```python
from build123d import *

# Parameters (mm, degrees)
F2_DEPTH = 2


# Not quite as in the source:
# - the program builds the solid bodies; features that only make, move or delete a surface that nothing else refers to are left out


with BuildPart() as f2:
    # F0 (on Top) → F2 (new body)
    with BuildSketch(Plane.XY):
        Polygon((-350, -225), (350, -225), (350, -217.2532975674), (350, 225), (-350, 225), align=None)
        with BuildLine():
            Line((197.5, 160), (197.5, -160))
            Line((197.5, -160), (-197.5, -160))
            Line((-197.5, -160), (-197.5, 84.3677148223))
            Line((-197.5, 84.3677148223), (-197.5, 160))
            Line((-197.5, 160), (-84.6111023318, 160))
            ThreePointArc((-84.6111023318, 160), (-82.6551501399, 160.0153039327), (-80.699197948, 160))
            Line((-80.699197948, 160), (197.5, 160))
        make_face(mode=Mode.SUBTRACT)
    extrude(amount=F2_DEPTH)


solid = f2.part
```
Input: part model. Units: mm. Frame: model coordinates. Give positions to 0.01 mm unless a question says otherwise; leave off trailing zeros. Order: outer loops, then holes, each group sorted by start corner. A loop starts at its lowest first (then second) coordinate and runs counter-clockwise, first axis right, second up. Notation, with made-up numbers: M -27.75,-30 L 20.25,-30 A18 cw 20.25,-8 Z; hole C -24,23 d10. An arc over 180 degrees is marked long. Return JSON: item names as keys, results as strings.
1) Section query A-A on y = 29. Output: boundary loops of the cut face in (x, z), and give its area (3 significant figures).
Taken from the geometry:
{"outline": "M -350,0 L -197.5,0 L -197.5,2 L -350,2 Z; M 197.5,0 L 350,0 L 350,2 L 197.5,2 Z", "area": "610 mm2"}
2) Section query C-C on x = 181. Output: boundary loops of the cut face in (y, z).
Taken from the geometry:
{"outline": "M -225,0 L -160,0 L -160,2 L -225,2 Z; M 160,0 L 225,0 L 225,2 L 160,2 Z"}
3) Section query B-B on z = 1.65. Output: boundary loops of the cut face in (x, y).
Taken from the geometry:
{"outline": "M -350,-225 L 350,-225 L 350,225 L -350,225 Z; hole M -197.5,-160 L 197.5,-160 L 197.5,160 L -80.7,160 A125 ccw -84.61,160 L -197.5,160 Z"}
4) Line query: L1, parallel to X at y = 1, z = 0.2; L2, parallel to Y at x = -64.5, z = 1.1. Output: solid intervals per line, ascending. Write a range as [from, to].
Taken from the geometry:
{"L1": "x = [-350, -197.5], [197.5, 350]", "L2": "y = [-225, -160], [160, 225]"}
